```python
from build123d import *

# Parameters (mm, degrees)
BOSS_EXTRUDE1_DEPTH   = 3
BOSS_EXTRUDE1_2_DEPTH = 3
BOSS_EXTRUDE1_3_DEPTH = 3
BOSS_EXTRUDE2_DEPTH   = 101.6
SKETCH2_R             = 6.000000000000007
SKETCH2_R_2           = 2.5526999999999953
SKETCH2_R_3           = 5.999999999999988
SKETCH2_R_4           = 2.5526999999999975
SKETCH2_R_5           = 6
SKETCH2_R_6           = 2.5527000000000024
SKETCH2_R_7           = 5.999999999999999
SKETCH2_R_8           = 2.552699999999999
SKETCH2_R_9           = 5.9999999999999964
SKETCH2_R_10          = 6.0000000000000036
SKETCH2_R_11          = 2.552700000000004
SKETCH2_R_12          = 2.5527000000000126
BOSS_EXTRUDE3_DEPTH   = 7.54
SKETCH2_3_R           = 2.5526999999999975
SKETCH2_3_R_2         = 2.5527000000000024
SKETCH2_3_R_3         = 2.552700000000004
SKETCH2_3_R_4         = 2.5527000000000126
SKETCH2_3_R_5         = 2.552699999999999
SKETCH2_3_R_6         = 2.5526999999999953
CUT_EXTRUDE1_DEPTH    = 143.3044492382441
SKETCH3_R             = 1.6499999999999975
SKETCH3_R_2           = 1.6500000000000021
CUT_EXTRUDE2_DEPTH    = 145.87603838454444
FILLET1_R             = 2.5399999999999996
FILLET2_R             = 2.5399999999999996
FILLET3_R             = 2.5399999999999996


with BuildPart() as part:
    # Sketch1 → Boss-Extrude1 (new body)
    with BuildSketch(Plane.XY):
        with BuildLine():
            Line((-58.198711325939165, 25.400000000000002), (-70.62855831036053, 25.400000000000002))
            ThreePointArc((-70.62855831036052, 25.39999999999999), (-74.61164899798933, 8.164256414446488), (-74.45016873050051, -9.524999999999999))
            Line((-74.45016873050054, -9.525), (-62.78156078818072, -9.525))
            ThreePointArc((-62.7815607881806, -9.524999999999148), (-62.96026895155072, 8.261630199203937), (-58.198711325939165, 25.4))
        make_face()
    extrude(amount=BOSS_EXTRUDE1_DEPTH)



with BuildPart() as body_2:
    # Sketch1 → Boss-Extrude1 2 (new body)
    with BuildSketch(Plane.XY):
        with BuildLine():
            Line((-61.48361062104342, -15.875), (-73.35896416935016, -15.875))
            ThreePointArc((-73.35896416935012, -15.874999999999993), (1.421e-14, -75.05699999999997), (73.35896416935014, -15.874999999999961))
            Line((73.35896416935016, -15.875), (61.48361062104344, -15.875))
            ThreePointArc((61.483610621043105, -15.874999999998629), (1.78e-15, -63.50000000000001), (-61.48361062104309, -15.874999999998634))
        make_face()
    extrude(amount=BOSS_EXTRUDE1_2_DEPTH)


with BuildPart() as body_3:
    # Sketch1 → Boss-Extrude1 3 (new body)
    with BuildSketch(Plane.XY):
        with BuildLine():
            ThreePointArc((58.19871132593919, 25.399999999999977), (62.96026895155074, 8.261630199203923), (62.78156078818061, -9.524999999999146))
            Line((62.78156078818074, -9.525), (74.45016873050054, -9.525))
            ThreePointArc((74.45016873050054, -9.524999999999999), (74.61164899798936, 8.164256414446513), (70.62855831036052, 25.400000000000006))
            Line((70.62855831036053, 25.400000000000002), (58.198711325939165, 25.400000000000002))
        make_face()
    extrude(amount=BOSS_EXTRUDE1_3_DEPTH)


with BuildPart() as part_1:
    add(part.part)

    add(body_2.part)  # Boss-Extrude2 merges body 2

    add(body_3.part)  # Boss-Extrude2 merges body 3
    # Sketch1_3 → Boss-Extrude2 (add)
    with BuildSketch(Plane.XY):
        with BuildLine():
            Line((-62.78156078818072, -9.525), (-74.45016873050054, -9.525))
            ThreePointArc((-74.45016873050051, -9.524999999999999), (-73.97273529586036, -12.711714355214593), (-73.35896416935012, -15.874999999999993))
            Line((-73.35896416935016, -15.875), (-61.48361062104342, -15.875))
            ThreePointArc((-61.48361062104309, -15.874999999998634), (-62.21365470168856, -12.71657063280289), (-62.7815607881806, -9.524999999999148))
        make_face()
        with BuildLine():
            Line((74.45016873050054, -9.525), (62.78156078818074, -9.525))
            ThreePointArc((62.78156078818061, -9.524999999999146), (62.213654701688576, -12.716570632802904), (61.483610621043105, -15.874999999998629))
            Line((61.48361062104344, -15.875), (73.35896416935016, -15.875))
            ThreePointArc((73.35896416935014, -15.874999999999991), (73.97273529586039, -12.711714355214575), (74.45016873050054, -9.524999999999999))
        make_face()
        with BuildLine():
            Line((62.78156078818074, -9.525), (-62.78156078818072, -9.525))
            ThreePointArc((-62.7815607881806, -9.524999999999148), (-62.21365470168856, -12.71657063280289), (-61.48361062104309, -15.874999999998634))
            Line((-61.48361062104342, -15.875), (61.48361062104344, -15.875))
            ThreePointArc((61.483610621043105, -15.874999999998629), (62.213654701688576, -12.716570632802904), (62.78156078818061, -9.524999999999146))
        make_face()
    extrude(amount=BOSS_EXTRUDE2_DEPTH)

    # Sketch2 → Boss-Extrude3 (add)
    # profile 1 of 8: a face of its own
    with BuildSketch(Plane(origin=(0, -9.525, 0), x_dir=(1, 0, 0), z_dir=(0, 1, 0))):
        with Locations(Location((-34.29, -63.5, 0), (0, 0, 270))):
            Circle(SKETCH2_R)
        with Locations(Location((-34.29, -63.5, 0), (0, 0, 270))):
            Circle(SKETCH2_R_2, mode=Mode.SUBTRACT)
    # profile 2 of 8: a face of its own
    with BuildSketch(Plane(origin=(0, -9.525, 0), x_dir=(1, 0, 0), z_dir=(0, 1, 0))):
        with Locations(Location((-34.29, -50.8, 0), (0, 0, 270))):
            Circle(SKETCH2_R_3)
        with Locations(Location((-34.29, -50.8, 0), (0, 0, 270))):
            Circle(SKETCH2_R_4, mode=Mode.SUBTRACT)
    # profile 3 of 8: a face of its own
    with BuildSketch(Plane(origin=(0, -9.525, 0), x_dir=(1, 0, 0), z_dir=(0, 1, 0))):
        with Locations(Location((-6.349999999999996, -50.8, 0), (0, 0, 270))):
            Circle(SKETCH2_R_5)
        with Locations(Location((-6.349999999999996, -50.8, 0), (0, 0, 270))):
            Circle(SKETCH2_R_6, mode=Mode.SUBTRACT)
    # profile 4 of 8: a face of its own
    with BuildSketch(Plane(origin=(0, -9.525, 0), x_dir=(1, 0, 0), z_dir=(0, 1, 0))):
        with Locations(Location((-6.349999999999996, -63.5, 0), (0, 0, 270))):
            Circle(SKETCH2_R_7)
        with Locations(Location((-6.349999999999996, -63.5, 0), (0, 0, 270))):
            Circle(SKETCH2_R_8, mode=Mode.SUBTRACT)
    # profile 5 of 8: a face of its own
    with BuildSketch(Plane(origin=(0, -9.525, 0), x_dir=(1, 0, 0), z_dir=(0, 1, 0))):
        with Locations(Location((6.350000000000014, -63.5, 0), (0, 0, 270))):
            Circle(SKETCH2_R_9)
        with Locations(Location((6.350000000000014, -63.5, 0), (0, 0, 270))):
            Circle(SKETCH2_R_8, mode=Mode.SUBTRACT)
    # profile 6 of 8: a face of its own
    with BuildSketch(Plane(origin=(0, -9.525, 0), x_dir=(1, 0, 0), z_dir=(0, 1, 0))):
        with Locations(Location((6.35000000000001, -50.8, 0), (0, 0, 270))):
            Circle(SKETCH2_R_7)
        with Locations(Location((6.35000000000001, -50.8, 0), (0, 0, 270))):
            Circle(SKETCH2_R_6, mode=Mode.SUBTRACT)
    # profile 7 of 8: a face of its own
    with BuildSketch(Plane(origin=(0, -9.525, 0), x_dir=(1, 0, 0), z_dir=(0, 1, 0))):
        with Locations(Location((34.29000000000001, -50.79999999999999, 0), (0, 0, 270))):
            Circle(SKETCH2_R_10)
        with Locations(Location((34.29000000000001, -50.79999999999999, 0), (0, 0, 270))):
            Circle(SKETCH2_R_11, mode=Mode.SUBTRACT)
    # profile 8 of 8: a face of its own
    with BuildSketch(Plane(origin=(0, -9.525, 0), x_dir=(1, 0, 0), z_dir=(0, 1, 0))):
        with Locations(Location((34.29000000000001, -63.499999999999986, 0), (0, 0, 270))):
            Circle(SKETCH2_R_10)
        with Locations(Location((34.29000000000001, -63.499999999999986, 0), (0, 0, 270))):
            Circle(SKETCH2_R_12, mode=Mode.SUBTRACT)
    extrude(amount=BOSS_EXTRUDE3_DEPTH)

    # Sketch2_3 → Cut-Extrude1 (cut, through all)
    with BuildSketch(Plane(origin=(0, -9.525, 0), x_dir=(1, 0, 0), z_dir=(0, 1, 0))):
        with Locations(Location((-34.29, -50.8, 0), (0, 0, 270))):
            Circle(SKETCH2_3_R)
        with Locations(Location((-6.349999999999996, -50.8, 0), (0, 0, 270))):
            Circle(SKETCH2_3_R_2)
        with Locations(Location((6.35000000000001, -50.8, 0), (0, 0, 270))):
            Circle(SKETCH2_3_R_2)
        with Locations(Location((34.29000000000001, -50.79999999999999, 0), (0, 0, 270))):
            Circle(SKETCH2_3_R_3)
        with Locations(Location((34.29000000000001, -63.499999999999986, 0), (0, 0, 270))):
            Circle(SKETCH2_3_R_4)
        with Locations(Location((6.350000000000014, -63.5, 0), (0, 0, 270))):
            Circle(SKETCH2_3_R_5)
        with Locations(Location((-6.349999999999996, -63.5, 0), (0, 0, 270))):
            Circle(SKETCH2_3_R_5)
        with Locations(Location((-34.29, -63.5, 0), (0, 0, 270))):
            Circle(SKETCH2_3_R_6)
    extrude(amount=-CUT_EXTRUDE1_DEPTH, mode=Mode.SUBTRACT)

    # Sketch3 → Cut-Extrude2 (cut, through all)
    with BuildSketch(Plane.XY.offset(3)):
        with Locations((0, -69.24071309920174)):
            Circle(SKETCH3_R)
        with Locations((69.24071309920174, 0)):
            Circle(SKETCH3_R_2)
        with Locations((-69.24071309920174, 0)):
            Circle(SKETCH3_R_2)
    extrude(amount=-CUT_EXTRUDE2_DEPTH, mode=Mode.SUBTRACT)

    # Fillet1
    fillet1_edges = [part_1.edges().sort_by_distance(p)[0] for p in [
        (58.198711325939186, 25.39999999999999, 1.5),
        (70.62855831036052, 25.400000000000002, 1.5),
        (-70.62855831036052, 25.4, 1.5),
        (-58.19871132593916, 25.4, 1.5),
    ]]
    fillet(fillet1_edges, radius=FILLET1_R)

    # Fillet2
    fillet2_edges = [part_1.edges().sort_by_distance(p)[0] for p in [
        (-68.61586475934062, -9.525, 3),
        (-67.42128739519679, -15.875, 3),
        (67.4212873951968, -15.875, 3),
        (68.61586475934064, -9.525, 3),
    ]]
    fillet(fillet2_edges, radius=FILLET2_R)

    # Fillet3
    fillet3_edges = [part_1.edges().sort_by_distance(p)[0] for p in [
        (62.781560788180585, -9.524999999999785, 2.7699999999999996),
        (61.48361062104301, -15.874999999999657, 2.7699999999999996),
        (-61.483610621043, -15.87499999999966, 2.7699999999999996),
        (-62.781560788180556, -9.524999999999785, 2.7699999999999996),
    ]]
    fillet(fillet3_edges, radius=FILLET3_R)


solid = part_1.part
```
Input: part model. Units: mm. Frame: model coordinates. A direction names the side the tool comes from. Round coordinates to 2 decimals unless told otherwise and drop trailing zeros. Loops run counter-clockwise (first coordinate to the right, second up) from the corner with the lowest first, then second, coordinate; pieces in that order, holes last. Notation, with made-up numbers: (7.25, -24) -> (16.25, -24) arc R11 ccw to (16.25, -9) -> close; hole circle Ø4 at (75.25, -28.5). An arc over 180 degrees is marked (long way). One line per item, written item: value.
(1) Section D-D (z = 92). Return the cut outline in (x, y) (3 decimals), plus the area to 3 significant figures.
Geometry check:
outline: (-74.45, -9.525) arc R75.057 ccw to (-73.359, -15.875) -> (73.359, -15.875) arc R75.057 ccw to (74.45, -9.525) -> close
area: 939 mm2
(2) Mould query, pull axis Y, two halves, no side actions, for faces 4 (the face through (-37, -1.985, 51)), 5 (the face through (59.831, -16.545, 2.193)), 6 (the face through (-5.7, -63.4, 3)). Classes: pulls with the +Y half, pulls with the -Y half, needs draft (parallel to the pull), parting line crosses it, or undercut.
Geometry check:
face 4: pulls with the +Y half
face 5: undercut
face 6: needs draft
(3) Pin query (flat end, axial travel): pin 1 (6.5 mm diameter, centred on x = -34.29, z = 63.5, fed in from -Y) (3 decimals); pin 2 (3 mm diameter, centred on x = 6.35, z = 50.8, fed in from +Y); pin 3 (3.5 mm diameter, centred on x = -31.5, z = 61, fed in from +Y) (3 decimals); pin 4 (1.5 mm diameter, centred on x = -54, z = 71.5, fed in from +Y) (3 decimals). Return the tip coordinate at first contact, or that it passes through.
Geometry check:
pin 1: y = -15.875
pin 2: through
pin 3: y = -1.985
pin 4: y = -9.525
(4) Section A-A (y = -26). Return the cut outline in (x, z).
Geometry check:
outline: (-70.41, 0) -> (-57.93, 0) -> (-57.93, 3) -> (-70.41, 3) -> close; (57.93, 0) -> (70.41, 0) -> (70.41, 3) -> (57.93, 3) -> close
(5) Material intervals for line 1 (Z direction, x = -6, y = -11); line 2 (X direction, y = -10.75, z = 63.5); line 3 (X direction, y = -13.25, z = 63.5), sorted ascending. Write a range as [from, to].
Geometry check:
line 1: [0, 48.27], [53.33, 60.97], [66.03, 101.6]
line 2: [-74.28, -36.84], [-31.74, -8.9], [-3.8, 3.8], [8.9, 31.74], [36.84, 74.28]
line 3: [-73.88, -36.84], [-31.74, -8.9], [-3.8, 3.8], [8.9, 31.74], [36.84, 73.88]
(6) Section B-B (x = 6.35). Return the cut outline in (y, z) (3 decimals).
Geometry check:
outline: (-74.788, 0) -> (-63.182, 0) -> (-63.182, 3) -> (-74.788, 3) -> close; (-15.875, 0) -> (-9.525, 0) -> (-9.525, 44.8) -> (-1.985, 44.8) -> (-1.985, 48.247) -> (-15.875, 48.247) -> close; (-15.875, 53.353) -> (-1.985, 53.353) -> (-1.985, 56.8) -> (-9.525, 56.8) -> (-9.525, 57.5) -> (-1.985, 57.5) -> (-1.985, 60.947) -> (-15.875, 60.947) -> close; (-15.875, 66.053) -> (-1.985, 66.053) -> (-1.985, 69.5) -> (-9.525, 69.5) -> (-9.525, 101.6) -> (-15.875, 101.6) -> close
(7) Section C-C (z = 63.5). Give the number of separate pieces and of enclosed holes in the cut face, plus the area to 3 significant figures.
Geometry check:
separate pieces: 5
enclosed holes: 0
area: 1,020 mm2
(8) Set-up query: faces 1 (the face through (-59.831, -16.545, 2.116)), 2 (the face through (4.05, -5.81, 56.34)), 3 (the face through (-1, -13, 101.6)). Return all of +Z, -Z, +X, -X, +Y, -Y with unobstructed straight access to the full face (end or side cutting, diameter ignored); none if empty.
Geometry check:
face 1: +Z, -Z
face 2: +Y
face 3: +Z, +X, -X, +Y, -Y
